Input: dimensioned drawing with shaded views. Units: mm. Origin: part minimum x, y, z. A direction names the side the tool comes from. Coordinates: 2 decimals unless noted, no trailing zeros. Order: outer loops, then holes, each group sorted by start corner. A loop starts at its lowest first (then second) coordinate and runs counter-clockwise, first axis right, second up. Notation, with made-up numbers: (13, 63) - (19, 63) arc R25 ccw to (19, 76) - close; hole circle Ø7 at (-15, 71). An arc over 180 degrees is marked (long way). Use one line per item in the form item = value. Start each with the question number.
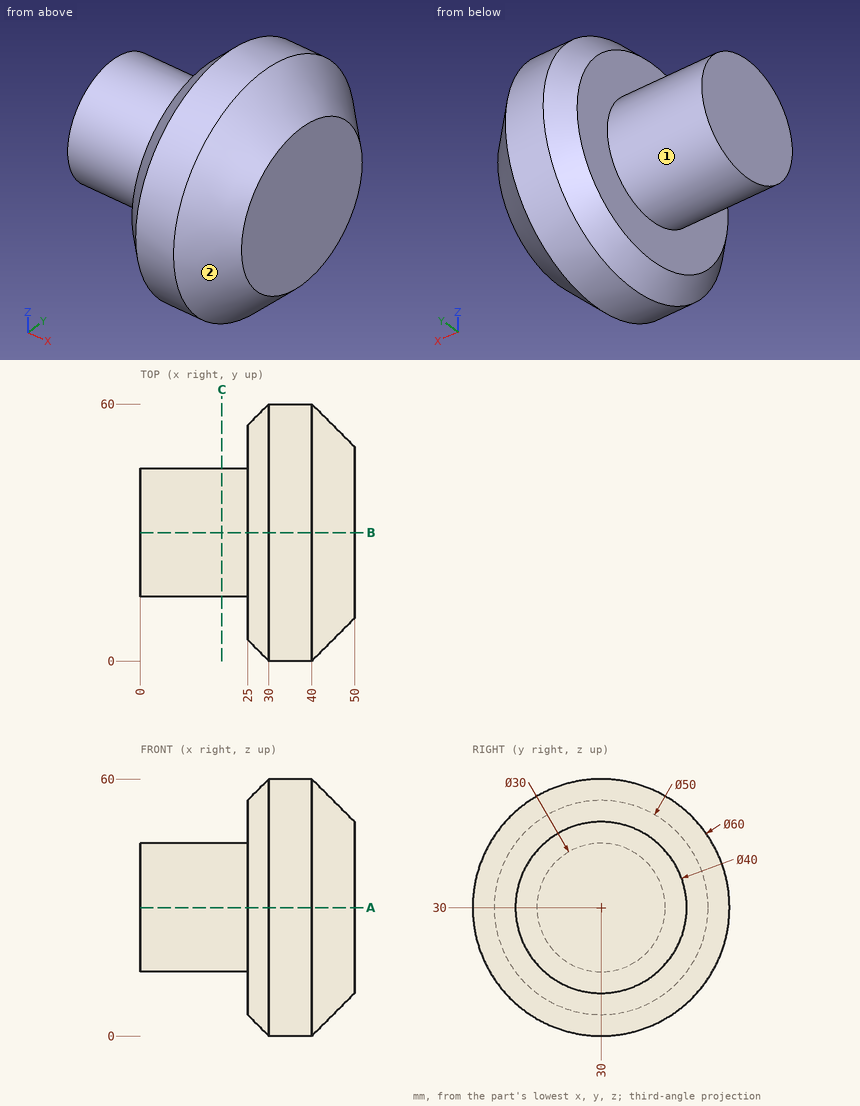
(1) Material intervals for L1, parallel to Z at x = 36.5, y = 30.5; L2, parallel to X at y = 49.5, z = 31; L3, parallel to Z at x = 9, y = 29.5, sorted ascending. Write a range as from..to.
(2) Cut plane A-A on z = 30. Return the cut outline in (x, y).
(3) Contact query for flat-ended pins moving along their axis: pin 1 Ø12 at (x, y) = (16.5, 29) entering from -Z; pin 2 Ø8 at (y, z) = (44, 13) entering from -X; pin 3 Ø12 at (x, y) = (31, 20) entering from +Z. Output: stop coordinate, or through.
(4) Cut plane C-C on x = 19. Return the cut outline in (y, z).
(5) Set-up query: the marked faces 1 and 2. Return all of +Z, -Z, +X, -X, +Y, -Y with unobstructed straight access to the full face (end or side cutting, diameter ignored); none if empty.
Check sheet entries:
q1.L1 = 0..60
q1.L2 = 25..50
q1.L3 = 15.01..44.99
q2.outline = (0, 15) - (25, 15) - (25, 5) - (30, 0) - (40, 0) - (50, 10) - (50, 50) - (40, 60) - (30, 60) - (25, 55) - (25, 45) - (0, 45) - close
q3.pin_1 = 15
q3.pin_2 = 25
q3.pin_3 = 59.73
q4.outline = circle Ø30 at (30, 30)
q5.face_1 = -X
q5.face_2 = +X
